```python
from build123d import *

# Parameters (mm, degrees)
SKETCH1_R           = 4.93
SKETCH1_R_2         = 2.75
BOSS_EXTRUDE1_DEPTH = 4.7625


with BuildPart() as part:
    # Sketch1 → Boss-Extrude1 (new body)
    with BuildSketch(Plane.XY):
        with BuildLine():
            Line((-85, 0), (85, 0))
            Line((85, 0), (85, 50))
            Line((85, 50), (65, 50))
            ThreePointArc((65, 50), (0, 30.871205009), (-65, 50))
            Line((-65, 50), (-85, 50))
            Line((-85, 50), (-85, 0))
        make_face()
        with Locations((0, 20)):
            Circle(SKETCH1_R, mode=Mode.SUBTRACT)
        with Locations((-75, 40)):
            Circle(SKETCH1_R_2, mode=Mode.SUBTRACT)
        with Locations((-75, 10)):
            Circle(SKETCH1_R_2, mode=Mode.SUBTRACT)
        with Locations((75, 40)):
            Circle(SKETCH1_R_2, mode=Mode.SUBTRACT)
        with Locations((75, 10)):
            Circle(SKETCH1_R_2, mode=Mode.SUBTRACT)
        with BuildLine():
            Line((-65, 28.82203459), (-65, 16))
            ThreePointArc((-65, 16), (-63.535533906, 12.464466094), (-60, 11))
            Line((-60, 11), (-29.111861318, 11))
            ThreePointArc((-29.111861318, 11), (-23.146216554, 16.358842801), (-27.836889289, 22.862972482))
            ThreePointArc((-27.836889289, 22.862972482), (-43.132909972, 27.17580462), (-57.794117647, 33.309136444))
            ThreePointArc((-57.794117647, 33.309136444), (-62.642970699, 33.066408028), (-65, 28.82203459))
        make_face(mode=Mode.SUBTRACT)
        with BuildLine():
            Line((65, 28.82203459), (65, 16))
            ThreePointArc((65, 16), (63.535533906, 12.464466094), (60, 11))
            Line((60, 11), (29.111861318, 11))
            ThreePointArc((29.111861318, 11), (23.146216554, 16.358842801), (27.836889289, 22.862972482))
            ThreePointArc((27.836889289, 22.862972482), (43.132909972, 27.17580462), (57.794117647, 33.309136444))
            ThreePointArc((57.794117647, 33.309136444), (62.642970699, 33.066408028), (65, 28.82203459))
        make_face(mode=Mode.SUBTRACT)
    extrude(amount=BOSS_EXTRUDE1_DEPTH)


solid = part.part
```
Geometry: final body of the model. Coordinates: model frame, mm. A direction names the side the tool comes from. Round coordinates to 2 decimals unless told otherwise and drop trailing zeros. Order: outer loops, then holes, each group sorted by start corner. A loop starts at its lowest first (then second) coordinate and runs counter-clockwise, first axis right, second up. Notation, with made-up numbers: M 69.5,4 L 112.5,4 A34 cw 112.5,37 Z; hole C 15.5,-19.75 d1. An arc over 180 degrees is marked long. Use one line per item in the form item = value. Start each with the question number.
Q1. Access query for faces 1 (the face through (-75, 50, 2)), 2 (the face through (-42.92, 27.1, 2.35)). Directions: +Z, -Z, +X, -X, +Y, -Y. A direction counts if a zero-diameter tool reaches every point of the face in a straight line with its end or side. Return the directions, or none.
Q2. Material intervals for line 1 (Y direction, x = 75, z = 3.75); line 2 (X direction, y = 12.5, z = 2.55); line 3 (Y direction, x = 0, z = 2.6), sorted ascending. Write a range as [from, to].
Q3. Cut plane C-C (z = 2.2). Return loops of the section in (x, y), and give its area (3 significant figures).
Q4. Pin query (flat end, axial travel): pin 1 Ø2 at (x, y) = (-0.5, 18) entering from +Z. Return the tip coordinate at first contact, or that it passes through.
Q5. Cut plane B-B (x = 0). Return loops of the section in (y, z), and give its area (3 significant figures).
Q6. Mould query, pull axis X, two halves, no side actions, for faces 3 (the face through (-62.582, 33.103, 2.348)), 4 (the face through (-1, 25, 0)). Classes: +X half, -X half, draft (parallel to the pull), parting line (faces both ways), or undercut.
Q7. Cut plane A-A (x = -75). Return loops of the section in (y, z), and give its area (3 significant figures).
Q8. Cut plane D-D (y = 40). Return loops of the section in (x, z), and give its area (3 significant figures).
Geometry results:
q1.face_1 = +Z, -Z, +X, -X, +Y
q1.face_2 = +Z, -Z
q2.line_1 = [0, 7.25], [12.75, 37.25], [42.75, 50]
q2.line_2 = [-85, -76.15], [-73.85, -63.57], [-25.14, 25.14], [63.57, 73.85], [76.15, 85]
q2.line_3 = [0, 15.07], [24.93, 30.87]
q3.outline = M -85,0 L 85,0 L 85,50 L 65,50 A120 cw -65,50 L -85,50 Z; hole C -75,10 d5.5; hole C -75,40 d5.5; hole M -65,16 A5 ccw -60,11 L -29.11,11 A6 ccw -27.84,22.86 A131 cw -57.79,33.31 A5 ccw -65,28.82 Z; hole C 0,20 d9.86; hole M 27.84,22.86 A6 ccw 29.11,11 L 60,11 A5 ccw 65,16 L 65,28.82 A5 ccw 57.79,33.31 A131 cw Z; hole C 75,10 d5.5; hole C 75,40 d5.5
q3.area = 5,270 mm^2
q4.pin_1 = through
q5.outline = M 0,0 L 15.07,0 L 15.07,4.76 L 0,4.76 Z; M 24.93,0 L 30.87,0 L 30.87,4.76 L 24.93,4.76 Z
q5.area = 100 mm^2
q6.face_3 = undercut
q6.face_4 = draft
q7.outline = M 0,0 L 7.25,0 L 7.25,4.76 L 0,4.76 Z; M 12.75,0 L 37.25,0 L 37.25,4.76 L 12.75,4.76 Z; M 42.75,0 L 50,0 L 50,4.76 L 42.75,4.76 Z
q7.area = 186 mm^2
q8.outline = M -85,0 L -77.75,0 L -77.75,4.76 L -85,4.76 Z; M -72.25,0 L -45.91,0 L -45.91,4.76 L -72.25,4.76 Z; M 45.91,0 L 72.25,0 L 72.25,4.76 L 45.91,4.76 Z; M 77.75,0 L 85,0 L 85,4.76 L 77.75,4.76 Z
q8.area = 320 mm^2
